```python
from build123d import *

# Parameters (mm, degrees)
EXTRUDE_1_DEPTH     = 20
SKETCH_2_R          = 25
EXTRUDE_2_DEPTH     = 10
SKETCH_5_W          = 5
SKETCH_5_H          = 5
CUT_EXTRUDE_2_DEPTH = 20
SKETCH_6_R          = 1.75
CUT_EXTRUDE_3_DEPTH = 10
SKETCH_7_R          = 1.75
CUT_EXTRUDE_4_DEPTH = 38


with BuildPart() as part:
    # 草图1 → 凸台-拉伸1 (new body)
    with BuildSketch(Plane.XY):
        Polygon((-15.5, 7.5), (-15.5, -7.5), (-7.5, -7.5), (-7.5, -17.5), (7.5, -17.5), (7.5, -7.5), (15.5, -7.5), (15.5, 7.5), (7.5, 7.5), (7.5, 17.5), (-7.5, 17.5), (-7.5, 7.5), align=None)
        Polygon((-10.5, 2.5), (-2.5, 2.5), (-2.5, 12.5), (2.5, 12.5), (2.5, 2.5), (10.5, 2.5), (10.5, -2.5), (2.5, -2.5), (2.5, -12.5), (-2.5, -12.5), (-2.5, -2.5), (-10.5, -2.5), align=None, mode=Mode.SUBTRACT)
    extrude(amount=EXTRUDE_1_DEPTH)

    # 草图2 → 凸台-拉伸2 (add)
    with BuildSketch(Plane.XY.offset(20)):
        Circle(SKETCH_2_R)
        Polygon((-10.5, -2.5), (-2.5, -2.5), (-2.5, -12.5), (2.5, -12.5), (2.5, -2.5), (10.5, -2.5), (10.5, 2.5), (2.5, 2.5), (2.5, 12.5), (-2.5, 12.5), (-2.5, 2.5), (-10.5, 2.5), align=None, mode=Mode.SUBTRACT)
    extrude(amount=EXTRUDE_2_DEPTH)

    # 草图5 → 切除-拉伸2 (cut)
    with BuildSketch(Plane(origin=(0, 0, 0), x_dir=(-1, 0, 0), z_dir=(0, 0, -1))):
        with Locations((0, 15)):
            Rectangle(SKETCH_5_W, SKETCH_5_H)
        with Locations((0, -15)):
            Rectangle(SKETCH_5_W, SKETCH_5_H)
    extrude(amount=-CUT_EXTRUDE_2_DEPTH, mode=Mode.SUBTRACT)

    # 草图6 → 切除-拉伸3 (cut)
    with BuildSketch(Plane(origin=(0, 0, 20), x_dir=(-1, 0, 0), z_dir=(0, 0, -1))):
        with Locations((14.849242405, 14.849242405)):
            Circle(SKETCH_6_R)
        with Locations((14.849242405, -14.849242405)):
            Circle(SKETCH_6_R)
        with Locations((-14.849242405, -14.849242405)):
            Circle(SKETCH_6_R)
        with Locations((-14.849242405, 14.849242405)):
            Circle(SKETCH_6_R)
    extrude(amount=-CUT_EXTRUDE_3_DEPTH, mode=Mode.SUBTRACT)

    # 草图7 → 切除-拉伸4 (cut)
    with BuildSketch(Plane.ZY.offset(7.5)):
        with Locations((10, 12.5)):
            Circle(SKETCH_7_R)
        with Locations((10, -12.5)):
            Circle(SKETCH_7_R)
    extrude(amount=-CUT_EXTRUDE_4_DEPTH, mode=Mode.SUBTRACT)


solid = part.part
```
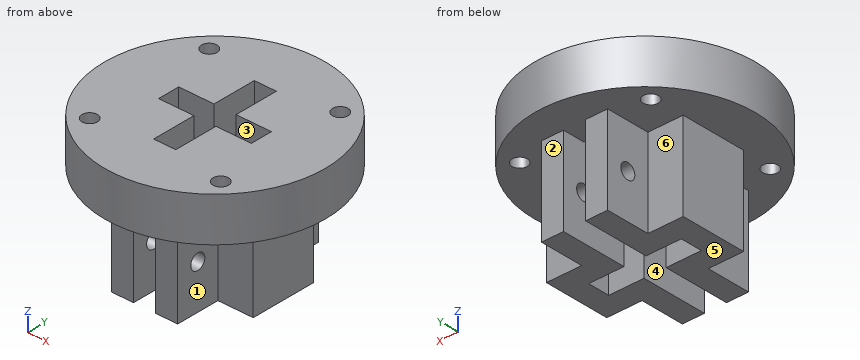
For this review, take the finished solid that the model builds, in its own axes (mm). Face numbers are marked on the shaded views. A direction names the side the tool comes from. Round coordinates to 2 decimals unless told otherwise and drop trailing zeros. Write each loop counter-clockwise with the first axis right and the second up, starting at its lowest first coordinate (ties: lowest second). Pieces come first, ordered by that corner, then holes. Notation, with made-up numbers: (8.25, 78.25) - (67.25, 78.25) arc R28 ccw to (67.25, 105.25) - close; hole circle Ø7 at (-33.75, -23). An arc over 180 degrees is marked (long way). Put each result on its own line as item: value.
Q1. We need section D-D (x = 0). Give the boundary of the cut face in (y, z).
Solved:
outline: (-25, 20) - (-12.5, 20) - (-12.5, 30) - (-25, 30) - close; (12.5, 20) - (25, 20) - (25, 30) - (12.5, 30) - close
Q2. We need section B-B (z = 18.25). Give the boundary of the cut face in (x, y).
Solved:
outline: (-15.5, -7.5) - (-7.5, -7.5) - (-7.5, -17.5) - (-2.5, -17.5) - (-2.5, -2.5) - (-10.5, -2.5) - (-10.5, 2.5) - (-2.5, 2.5) - (-2.5, 17.5) - (-7.5, 17.5) - (-7.5, 7.5) - (-15.5, 7.5) - close; (2.5, -17.5) - (7.5, -17.5) - (7.5, -7.5) - (15.5, -7.5) - (15.5, 7.5) - (7.5, 7.5) - (7.5, 17.5) - (2.5, 17.5) - (2.5, 2.5) - (10.5, 2.5) - (10.5, -2.5) - (2.5, -2.5) - close
Q3. Mouldability with a two-part tool opening along Y and no side actions: class the marked faces 4, 5 and 6 as released by +Y, released by -Y, zero draft, split by the parting line, or undercut.
Solved:
face 4: undercut
face 5: zero draft
face 6: released by +Y
Q4. Insertion check: pin 1 Ø4 at (x, z) = (-1, 4) entering from +Y; pin 2 Ø11 at (y, z) = (-11.5, 11) entering from +X; pin 3 Ø4 at (x, y) = (-14.85, -14.85) entering from -Z. Each pin has a flat end and moves straight along its axis. Give the tip position at first contact, or say it passes through.
Solved:
pin 1: stops at y = 17.5
pin 2: stops at x = 15.5
pin 3: stops at z = 20
Q5. We need section C-C (x = 6.5). Give the boundary of the cut face in (y, z).
Solved:
outline: (-24.14, 20) - (-17.5, 20) - (-17.5, 0) - (-2.5, 0) - (-2.5, 30) - (-24.14, 30) - close; (2.5, 0) - (17.5, 0) - (17.5, 20) - (24.14, 20) - (24.14, 30) - (2.5, 30) - close; hole circle Ø3.5 at (-12.5, 10); hole circle Ø3.5 at (12.5, 10)
Q6. We need section A-A (y = 0). Give the boundary of the cut face in (x, z), and give its area (3 significant figures).
Solved:
outline: (-25, 20) - (-15.5, 20) - (-15.5, 0) - (-10.5, 0) - (-10.5, 30) - (-25, 30) - close; (10.5, 0) - (15.5, 0) - (15.5, 20) - (25, 20) - (25, 30) - (10.5, 30) - close
area: 490 mm2
Q7. Machinability: for the marked faces 1, 2 and 3, which of the approach directions +Z, -Z, +X, -X, +Y, -Y give a long, thin tool a straight path to every point of the face, cutting with its end or side? Answer none if there is none.
Solved:
face 1: -Z, +X, -Y
face 2: -Z, +X, -X, +Y
face 3: +Z, -Z
Q8. Wall thickness on probe 1 along X at (y, z) = (-13, 18.75); probe 2 along Y at (x, z) = (-4.45, 10): over which ranges is each line inside the solid? List them lowest first.
Solved:
probe 1: x = -7.5 to -2.5, 2.5 to 7.5
probe 2: y = -17.5 to -14.25, -10.75 to -2.5, 2.5 to 10.75, 14.25 to 17.5
